```python
from build123d import *

# Parameters (mm, degrees)
IZIM1_W                     = 10.606601718
IZIM1_H                     = 10.606601718
Y_KSEKLIK_EKSTR_ZYON1_DEPTH = 2
IZIM2_R                     = 3.95
Y_KSEKLIK_EKSTR_ZYON2_DEPTH = 55
KES_EKSTR_ZYON1_DEPTH       = 10
IZIM5_R                     = 1.6
KES_EKSTR_ZYON3_DEPTH       = 26
IZIM8_W                     = 5
IZIM8_H                     = 13.621024602
KES_EKSTR_ZYON4_DEPTH       = 58.49130369


with BuildPart() as part:
    # Çizim1 → Yükseklik-Ekstrüzyon1 (new body)
    with BuildSketch(Plane.XY):
        Rectangle(IZIM1_W, IZIM1_H)
    extrude(amount=Y_KSEKLIK_EKSTR_ZYON1_DEPTH)

    # Çizim2 → Yükseklik-Ekstrüzyon2 (add)
    with BuildSketch(Plane(origin=(0, 0, 0), x_dir=(-1, 0, 0), z_dir=(0, 0, -1))):
        with Locations(Location((0, 0, 0), (0, 0, 180))):
            Circle(IZIM2_R)
    extrude(amount=Y_KSEKLIK_EKSTR_ZYON2_DEPTH)

    # Çizim3 → Kes-Ekstrüzyon1 (cut)
    with BuildSketch(Plane.XY.offset(2)):
        with BuildLine():
            Line((-2, -1.959591794), (-2, 1.959591794))
            ThreePointArc((-2, 1.959591794), (0, 2.8), (2, 1.959591794))
            Line((2, 1.959591794), (2, -1.959591794))
            ThreePointArc((2, -1.959591794), (0, -2.8), (-2, -1.959591794))
        make_face()
    extrude(amount=-KES_EKSTR_ZYON1_DEPTH, mode=Mode.SUBTRACT)

    # Çizim5 → Kes-Ekstrüzyon3 (cut, symmetric)
    with BuildSketch(Plane(origin=(0, 0, 0), x_dir=(0, 0, -1), z_dir=(1, 0, 0))):
        with Locations((29.6, 0)):
            Circle(IZIM5_R)
        with Locations((47.6, 0)):
            Circle(IZIM5_R)
    extrude(amount=KES_EKSTR_ZYON3_DEPTH, both=True, mode=Mode.SUBTRACT)

    # Çizim8 → Kes-Ekstrüzyon4 (cut, through all)
    with BuildSketch(Plane(origin=(0, 0, -55), x_dir=(-1, 0, 0), z_dir=(0, 0, -1))):
        with Locations((-5.8, 0)):
            Rectangle(IZIM8_W, IZIM8_H)
    extrude(amount=-KES_EKSTR_ZYON4_DEPTH, mode=Mode.SUBTRACT)


solid = part.part
```
Verification items for the finished model (mm, model axes). A direction names the side the tool comes from. Give positions to 0.01 mm unless a question says otherwise; leave off trailing zeros. Order: outer loops, then holes, each group sorted by start corner. A loop starts at its lowest first (then second) coordinate and runs counter-clockwise, first axis right, second up. Notation, with made-up numbers: (10.5, 59.5) - (38.5, 59.5) arc R9 cw to (38.5, 75.5) - close; hole circle Ø10 at (-15.75, -18.75). An arc over 180 degrees is marked (long way). Answer as CSV lines item,"result". Start each with the question number.
Item 1: Section check B-B, the plane x = 2.75. Record the boundary of the cut face in (y, z), plus the area to 3 significant figures.
Item 2: Mould release check, pull along X, two halves, no side actions. Record for faces 1 (the face through (-1, -5.303, 1)), 2 (the face through (-3.947, -0.142, -27.115)), 3 (the face through (0, -2.8, -2.9)): released by +X, released by -X, zero draft, split by the parting line, or undercut.
Item 3: Material ranges on L1, parallel to Z at x = -3, y = 0; L2, parallel to Z at x = 1.7, y = 0; L3, parallel to Y at x = 0, z = -47.6, recorded low to high.
Item 4: Section check A-A, the plane y = 0. Record the boundary of the cut face in (x, z), plus the area to 3 significant figures.
Item 5: Access from +Z, -Z, +X, -X, +Y, -Y to the whole of each face (thin tool, end or side, straight path). Record for faces 4 (the face through (0, 0, -55)), 5 (the face through (-2, 0, -3)).
Item 6: Section check D-D, the plane z = -7. Record the boundary of the cut face in (x, y), plus the area to 3 significant figures.
Item 7: Section check C-C, the plane z = -29.6. Record the boundary of the cut face in (x, y).
Item 8: Gauge pin test, flat ends, axial feed: pin 1 (1.2 mm diameter, centred on y = 0.5, z = -3, fed in from -X); pin 2 (5 mm diameter, centred on y = 0, z = -29.6, fed in from -X); pin 3 (1 mm diameter, centred on x = -3.5, z = -23, fed in from -Y). Record the tip position at first contact, or that the pin passes through.
Filled in:
1,outline,"(-5.3, 0) - (-2.84, 0) - (-2.84, -55) - (2.84, -55) - (2.84, 0) - (5.3, 0) - (5.3, 2) - (-5.3, 2) - close; hole circle Ø3.2 at (0, -47.6); hole circle Ø3.2 at (0, -29.6)"
1,area,"317 mm^2"
2,face 1,"zero draft"
2,face 2,"split by the parting line"
2,face 3,"undercut"
3,L1,"-55 to -49.2, -46 to -31.2, -28 to 2"
3,L2,"-55 to -49.2, -46 to -31.2, -28 to -8"
3,L3,"-3.95 to -1.6, 1.6 to 3.95"
4,outline,"(-5.3, 0) - (-3.95, 0) - (-3.95, -28) - (3.3, -28) - (3.3, 2) - (2, 2) - (2, -8) - (-2, -8) - (-2, 2) - (-5.3, 2) - close; (-3.95, -55) - (3.3, -55) - (3.3, -49.2) - (-3.95, -49.2) - close; (-3.95, -46) - (3.3, -46) - (3.3, -31.2) - (-3.95, -31.2) - close"
4,area,"330 mm^2"
5,face 4,"-Z, +X, -X, +Y, -Y"
5,face 5,"+Z"
6,outline,"(3.3, -2.17) - (3.3, 2.17) arc R3.95 ccw (long way) to start; hole (-2, -1.96) arc R2.8 ccw to (2, -1.96) - (2, 1.96) arc R2.8 ccw to (-2, 1.96) - close"
6,area,"26.8 mm^2"
7,outline,"(-3.61, -1.6) arc R3.95 ccw to (3.3, -2.17) - (3.3, -1.6) - close; (-3.61, 1.6) - (3.3, 1.6) - (3.3, 2.17) arc R3.95 ccw to start"
8,pin 1,"x = -3.95"
8,pin 2,"x = -3.95"
8,pin 3,"y = -2.57"
